```python
from build123d import *

# Parameters (mm, degrees)
BOSS_EXTRUDE1_DEPTH                = 188.45
SKETCH6_W                          = 188.45
SKETCH6_H                          = 3
BOSS_EXTRUDE2_DEPTH                = 10
SKETCH7_W                          = 13
SKETCH7_H                          = 188.45
BOSS_EXTRUDE3_DEPTH                = 4
SKETCH8_W                          = 3
SKETCH8_H                          = 188.45
BOSS_EXTRUDE4_DEPTH                = 10
SKETCH9_W                          = 188.45
SKETCH9_H                          = 13
BOSS_EXTRUDE5_DEPTH                = 4
CSK_FOR_M3_SFHCS1_D                = 3.2
CSK_FOR_M3_SFHCS1_CSINK_D          = 6.72
CSK_FOR_M3_SFHCS1_CSINK_ANGLE      = 90
CSK_FOR_M3_SFHCS2_D                = 3.2
CSK_FOR_M3_SFHCS2_CSINK_D          = 6.72
CSK_FOR_M3_SFHCS2_CSINK_ANGLE      = 90
FILLET1_R                          = 1.5
F_4_4_4_4_DIAMETER_HOLE1_D         = 4.4
F_4_4_4_4_DIAMETER_HOLE1_DEPTH     = 10
F_4_4_4_4_DIAMETER_HOLE1_TIP       = 1.321893362
F_4_4_4_4_DIAMETER_HOLE3_D         = 4.4
F_4_4_4_4_DIAMETER_HOLE3_DEPTH     = 10
F_4_4_4_4_DIAMETER_HOLE3_TIP       = 1.321893362
SKETCH18_W                         = 12
SKETCH18_H                         = 24
CUT_EXTRUDE1_DEPTH                 = 2
F_4_3_START                        = -5
F_4_3_4_3_DIAMETER_HOLE1_OUTLINE_R = 2.15
F_4_3_4_3_DIAMETER_HOLE1_DEPTH     = 3
SKETCH21_W                         = 24
SKETCH21_H                         = 12
CUT_EXTRUDE2_DEPTH                 = 2
F_4_3_4_3_DIAMETER_HOLE2_OUTLINE_R = 2.15
F_4_3_4_3_DIAMETER_HOLE2_DEPTH     = 3


# Read off the part's stored shape, not the designer's step: Ø4.3 (4.3) Diameter Hole1, Ø4.3 (4.3) Diameter Hole2
with BuildPart() as part:
    # Sketch1 → Boss-Extrude1 (new body)
    with BuildSketch(Plane.XY.offset(280)):
        Polygon((-7, 4), (4, -7), (7, -7), (7, -3), (20, -3), (20, 0), (0, 0), (0, 20), (-3, 20), (-3, 7), (-7, 7), align=None)
    extrude(amount=-BOSS_EXTRUDE1_DEPTH)

    # Sketch6 → Boss-Extrude2 (add)
    with BuildSketch(Plane(origin=(20, 0, 0), x_dir=(0, 0, -1), z_dir=(1, 0, 0))):
        with Locations((-185.775, -1.5)):
            Rectangle(SKETCH6_W, SKETCH6_H)
    extrude(amount=BOSS_EXTRUDE2_DEPTH)

    # Sketch7 → Boss-Extrude3 (add)
    with BuildSketch(Plane.XZ.offset(3)):
        with Locations((13.5, 185.775)):
            Rectangle(SKETCH7_W, SKETCH7_H)
    extrude(amount=BOSS_EXTRUDE3_DEPTH)

    # Sketch8 → Boss-Extrude4 (add)
    with BuildSketch(Plane(origin=(0, 20, 0), x_dir=(1, 0, 0), z_dir=(0, 1, 0))):
        with Locations((-1.5, -185.775)):
            Rectangle(SKETCH8_W, SKETCH8_H)
    extrude(amount=BOSS_EXTRUDE4_DEPTH)

    # Sketch9 → Boss-Extrude5 (add)
    with BuildSketch(Plane.ZY.offset(3)):
        with Locations((185.775, 13.5)):
            Rectangle(SKETCH9_W, SKETCH9_H)
    extrude(amount=BOSS_EXTRUDE5_DEPTH)

    # CSK for M3 SFHCS1 (through all)
    with Locations(Plane.XZ.offset(7)):
        with Locations((10, 270)):
            CounterSinkHole(CSK_FOR_M3_SFHCS1_D / 2, CSK_FOR_M3_SFHCS1_CSINK_D / 2, counter_sink_angle=CSK_FOR_M3_SFHCS1_CSINK_ANGLE)

    # CSK for M3 SFHCS2 (through all)
    with Locations(Plane.ZY.offset(7)):
        with Locations((270, 10)):
            CounterSinkHole(CSK_FOR_M3_SFHCS2_D / 2, CSK_FOR_M3_SFHCS2_CSINK_D / 2, counter_sink_angle=CSK_FOR_M3_SFHCS2_CSINK_ANGLE)

    # Fillet1
    fillet1_edges = [part.edges().sort_by_distance(p)[0] for p in [
        (4, -7, 185.775),
        (-7, 4, 185.775),
    ]]
    fillet(fillet1_edges, radius=FILLET1_R)

    # Ø4.4 (4.4) Diameter Hole1
    with Locations(Plane.ZY.offset(3)):
        with Locations((185.775, 25)):
            Hole(F_4_4_4_4_DIAMETER_HOLE1_D / 2, depth=F_4_4_4_4_DIAMETER_HOLE1_DEPTH)
            with Locations((0, 0, -(F_4_4_4_4_DIAMETER_HOLE1_DEPTH + F_4_4_4_4_DIAMETER_HOLE1_TIP / 2))):  # 118° drill point
                Cone(0, F_4_4_4_4_DIAMETER_HOLE1_D / 2, F_4_4_4_4_DIAMETER_HOLE1_TIP, mode=Mode.SUBTRACT)

    # Ø4.4 (4.4) Diameter Hole3
    with Locations(Plane.XZ.offset(3)):
        with Locations((25, 185.775)):
            Hole(F_4_4_4_4_DIAMETER_HOLE3_D / 2, depth=F_4_4_4_4_DIAMETER_HOLE3_DEPTH)
            with Locations((0, 0, -(F_4_4_4_4_DIAMETER_HOLE3_DEPTH + F_4_4_4_4_DIAMETER_HOLE3_TIP / 2))):  # 118° drill point
                Cone(0, F_4_4_4_4_DIAMETER_HOLE3_D / 2, F_4_4_4_4_DIAMETER_HOLE3_TIP, mode=Mode.SUBTRACT)

    # Sketch18 → Cut-Extrude1 (cut)
    with BuildSketch(Plane(origin=(0, 0, 0), x_dir=(1, 0, 0), z_dir=(0, 1, 0))):
        with Locations((10, -103.55)):
            Rectangle(SKETCH18_W, SKETCH18_H)
    extrude(amount=-CUT_EXTRUDE1_DEPTH, mode=Mode.SUBTRACT)

    # Ø4.3 (4.3) Diameter Hole1 outline → Ø4.3 (4.3) Diameter Hole1 (cut)
    with BuildSketch(Plane(origin=(0, 0, 0), x_dir=(1, 0, 0), z_dir=(0, 1, 0)).offset(F_4_3_START)):
        with Locations((10, -109.55)):
            Circle(F_4_3_4_3_DIAMETER_HOLE1_OUTLINE_R)
        with Locations((10, -97.55)):
            Circle(F_4_3_4_3_DIAMETER_HOLE1_OUTLINE_R)
    extrude(amount=F_4_3_4_3_DIAMETER_HOLE1_DEPTH, mode=Mode.SUBTRACT)

    # Sketch21 → Cut-Extrude2 (cut)
    with BuildSketch(Plane(origin=(0, 0, 0), x_dir=(0, 0, -1), z_dir=(1, 0, 0))):
        with Locations((-103.55, 10)):
            Rectangle(SKETCH21_W, SKETCH21_H)
    extrude(amount=-CUT_EXTRUDE2_DEPTH, mode=Mode.SUBTRACT)

    # Ø4.3 (4.3) Diameter Hole2 outline → Ø4.3 (4.3) Diameter Hole2 (cut)
    with BuildSketch(Plane.YZ.offset(F_4_3_START)):
        with Locations((10, 109.55)):
            Circle(F_4_3_4_3_DIAMETER_HOLE2_OUTLINE_R)
        with Locations((10, 97.55)):
            Circle(F_4_3_4_3_DIAMETER_HOLE2_OUTLINE_R)
    extrude(amount=F_4_3_4_3_DIAMETER_HOLE2_DEPTH, mode=Mode.SUBTRACT)


solid = part.part
```
Model file for the job. Use its own axes, mm. A direction names the side the tool comes from. Round coordinates to 2 decimals unless told otherwise and drop trailing zeros. Loops run counter-clockwise (first coordinate to the right, second up) from the corner with the lowest first, then second, coordinate; pieces in that order, holes last. Notation, with made-up numbers: M 39.25,54 L 64.25,54 A19 ccw 64.25,90 Z; hole C 53,88 d4. An arc over 180 degrees is marked long. Put each result on its own line as item: value. Start each with the question number.
Item 1: Cut at A-A (x = 25). List the corners of the cut face in (y, z) (3 decimals), then the cut area to 3 significant figures.
Item 2: 3-axis set-ups, long thin cutter, end or side, ignore diameter. For faces 1 (the face through (-5, 10, 110)), 2 (the face through (-5, 20, 184)), 3 (the face through (-2, 10, 104)), 4 (the face through (10, -5, 110)): which of +Z, -Z, +X, -X, +Y, -Y reach the whole face in a straight line?
Item 3: Drill centre lines: line 1 along Z through (x, y) = (-4.15, 10); line 2 along Z through (x, y) = (10, -1.2); line 3 along X through (y, z) = (25, 204). Where is each one in solid material? Low to high.
Item 4: Cut at C-C (z = 270). List the corners of the cut face in (x, y), then the cut area to 3 significant figures.
Item 5: Drop flat-ended pins along their axis: P1, Ø5, axis at y = 10, z = 270, coming from the +X side; P2, Ø4.5, axis at y = 10, z = 109, coming from the +X side; P3, Ø11, axis at y = 23, z = 149, coming from the -X side; P4, Ø3.5, axis at x = 10.5, z = 109.5, coming from the +Y side. Give the stop position or say it passes through.
Item 6: Mould opens along Y. For faces 5 (the face through (-5, 10, 98)), 6 (the face through (25.286, -1.479, 187.956)), 7 (the face through (12, -7, 187)), 8 (the face through (10, -5, 98)) say: released by +Y, released by -Y, zero draft, split by the parting line, or undercut.
Answer block:
1. outline: M -3,91.55 L 0,91.55 L 0,183.575 L -3,183.575 Z; M -3,187.975 L 0,187.975 L 0,280 L -3,280 Z
1. area: 552 mm2
2. face 1: +X
2. face 2: +Z, -Z, -X, +Y
2. face 3: -Z, +X
2. face 4: +Y
3. line 1: 91.55 to 95.4, 99.7 to 107.4, 111.7 to 268.4, 271.6 to 280
3. line 2: 115.55 to 268.4, 271.6 to 280
3. line 3: -3 to 0
4. outline: M -7,4.62 A1.5 ccw -6.56,3.56 L 3.56,-6.56 A1.5 ccw 4.62,-7 L 6.64,-7 L 8.4,-5.24 L 8.4,0 L 0,0 L 0,8.4 L -5.24,8.4 L -7,6.64 Z; M -7,13.36 L -5.24,11.6 L 0,11.6 L 0,30 L -3,30 L -3,20 L -7,20 Z; M 11.6,-5.24 L 13.36,-7 L 20,-7 L 20,-3 L 30,-3 L 30,0 L 11.6,0 Z
4. area: 277 mm2
5. P1: x = 0
5. P2: x = -2
5. P3: x = -7
5. P4: y = -2
6. face 5: undercut
6. face 6: zero draft
6. face 7: released by -Y
6. face 8: released by +Y
